from build123d import *

# Parameters (mm, degrees)
F1_DEPTH = 5.08
F4_DEPTH = 5.08
F7_DEPTH = 5.08


with BuildPart() as f1:
    # F0 (on Front) → F1 (new body)
    with BuildSketch(Plane.XZ):
        Polygon((49.2544993758, 7.0634965241), (49.2544956505, 10.4342158884), (-41.1312952638, 10.4342158884), (-69.9499547482, 27.4472031742), (-71.8305518383, 24.2616199337), (-42.6982863529, 7.0634965241), align=None)
    extrude(amount=F1_DEPTH)


with BuildPart() as f4:
    # F3 (on Front) → F4 (new body)
    with BuildSketch(Plane.XZ):
        Polygon((-31.1960466206, 8.5284151137), (64.4119828939, 8.5284151137), (63.5142549872, 13.9479198755), (-31.1960466206, 13.9479198755), (-66.7409883864, -2.9896041492), (-64.6364092827, -7.406255696), align=None)
    extrude(amount=F4_DEPTH)


with BuildPart() as f7:
    # F6 (on Front) → F7 (new body)
    with BuildSketch(Plane.XZ):
        Polygon((61.6721026599, 7.6853110745), (61.6721026599, 10.9154162928), (-42.2426611185, 10.9154162928), (-75.4255279899, -7.6407911256), (-74.0495196081, -10.1014180153), (-42.2426611185, 7.6853110745), align=None)
    extrude(amount=F7_DEPTH)


solid = f7.part
Can you work these out from the model? Positions are in its coordinate system, mm. A direction names the side the tool comes from. Give positions to 0.01 mm unless a question says otherwise; leave off trailing zeros. Order: outer loops, then holes, each group sorted by start corner. A loop starts at its lowest first (then second) coordinate and runs counter-clockwise, first axis right, second up. Notation, with made-up numbers: M 72.25,75.25 L 111.25,75.25 A20 ccw 111.25,84.25 Z; hole C 23,70 d6. An arc over 180 degrees is marked long. Use a Markdown table: item, result. Add a question column.
Item 1: Suppose I cut it at A-A (y = -2). List the corners of the cut face in (x, z) for me.
Item 2: Suppose I cut it at B-B (x = 16). List the corners of the cut face in (y, z) for me, then the cut area to 3 significant figures.
Item 3: If I drill on L1, parallel to Z at x = 53, y = -1.1; L2, parallel to X at y = -1.5, z = -8.75; L3, parallel to X at y = -1.45, z = -6.75, over which ranges is the centre line in solid material (lowest first)? Write a range as [from, to].
Item 4: Suppose I cut it at C-C (z = 0.5). List the corners of the cut face in (x, y) for me, then the cut area to 3 significant figures.
Item 5: For faces 1 (the flat face through (9, -3, 7.685)), 2 (the flat face through (-7, 0, 9)), which set-ups out of +Z, -Z, +X, -X, +Y, -Y let a thin tool reach every point of the face, with its end or its side?
Item 6: Will these pins go through, and if not, where does the flat tip stop? pin 1 (2.5 mm diameter, centred on x = 16, y = -2.5, fed in from -Z); pin 2 (2 mm diameter, centred on y = -4, z = -3, fed in from +X); pin 3 (12 mm diameter, centred on x = -4.5, z = 5, fed in from -Y).
Answer sheet:
| question | item | result |
|---|---|---|
| 1 | outline | M -75.43,-7.64 L -74.05,-10.1 L -42.24,7.69 L 61.67,7.69 L 61.67,10.92 L -42.24,10.92 Z |
| 2 | outline | M -5.08,7.69 L 0,7.69 L 0,10.92 L -5.08,10.92 Z |
| 2 | area | 16.4 mm² |
| 3 | L1 | z = [7.69, 10.92] |
| 3 | L2 | x = [-74.81, -71.63] |
| 3 | L3 | x = [-73.83, -68.06] |
| 4 | outline | M -60.87,-5.08 L -55.09,-5.08 L -55.09,0 L -60.87,0 Z |
| 4 | area | 29.3 mm² |
| 5 | face 1 | -Z, +X, +Y, -Y |
| 5 | face 2 | +Z, -Z, +X, -X, +Y |
| 6 | pin 1 | stops at z = 7.69 |
| 6 | pin 2 | stops at x = -59.56 |
| 6 | pin 3 | stops at y = -5.08 |
